Model file for the job. Use its own axes, mm. Face numbers are marked on the shaded views. A direction names the side the tool comes from. Round coordinates to 2 decimals unless told otherwise and drop trailing zeros. Order: outer loops, then holes, each group sorted by start corner. A loop starts at its lowest first (then second) coordinate and runs counter-clockwise, first axis right, second up. Notation, with made-up numbers: (67, -33.5) -> (119, -33.5) arc R21 ccw to (119, -11.5) -> close; hole circle Ø10 at (-18, 3). An arc over 180 degrees is marked (long way). Use CSV: the item, a comma, the result in double quotes.
Autodesk Inventor part; units mm, degrees
ref_plane "Work Plane1" through (-7, 0, 0) normal (-1, 0, 0) x (0, 0, 1)
ref_plane "Work Plane2" through (-7, 0, -17.9) normal (0, -1, 0) x (1, 0, 0)
ref_plane "YZ Plane" through (0, 0, 0) normal (1, 0, 0) x (0, 1, 0)
sketch "Sketch1" plane through (0, 0, 0) normal (1, 0, 0) x (0, 1, 0)
  arc A0 (-3.4641, 2) -> (3.4641, 2) centre (0, 0) ccw
  arc A1 (-5.1962, 3) -> (5.1962, 3) centre (0, 0) ccw
  arc A2 (5.1962, 3) -> (3.4641, 2) centre (4.3301, 2.5) ccw
  arc A3 (-3.4641, 2) -> (-5.1962, 3) centre (-4.3301, 2.5) ccw
  dimension "d0" = 8
  dimension "d1" = 12
  dimension "d2" = 2.5
extrude "Extrusion1" add sketch "Sketch1" along normal blind 16
sketch "Sketch4" plane through (16, 0, 0) normal (1, 0, 0) x (0, 0, -1)
  point P0 (0, 0)
sketch "Sketch5" plane through (16, 0, 0) normal (1, 0, 0) x (0, 0, -1)
  line L0 (-6.2503, -10.1933) -> (7.7655, -10.1933)
  line L1 (7.7655, -10.1933) -> (7.7655, 0)
  line L2 (7.7655, 0) -> (-6.2503, 0)
  line L3 (-6.2503, 0) -> (-6.2503, -10.1933)
  point P0 (0, 0)
extrude "Extrusion4" cut sketch "Sketch5" against normal blind 3
ref_plane "Work Plane1" through (-7, 0, 0) normal (-1, 0, 0) x (0, 0, 1)
sketch "Sketch9" plane through (-7, 0, 0) normal (-1, 0, 0) x (0, 0, 1)
  line L0 (-17.9, 10) -> (-11.4, 10)
  line L1 (-11.4, 10) -> (-11.4, -10)
  line L2 (-11.4, -10) -> (-17.9, -10)
  line L3 (-17.9, -10) -> (-17.9, 10)
  point P0 (0, 0)
  point P1 (-17.9, 0)
  dimension "d34" = 11.4
  dimension "d35" = 6.5
  dimension "d36" = 20
extrude "Extrusion8" add sketch "Sketch9" along normal blind 5
ref_plane "Work Plane2" through (-7, 0, -17.9) normal (0, -1, 0) x (1, 0, 0)
sketch "Sketch10" plane through (-7, 0, -17.9) normal (0, -1, 0) x (1, 0, 0)
  line L0 (7, 11) -> (23, 11)
  line L1 (0, 0) -> (0, 6.5)
  line L2 (7, 11.9) -> (0, 6.5)
  line L3 (0, 0) -> (-5, 0)
  line L4 (0, 6.5) -> (0, 0)
  line L5 (0, 0) -> (15.4259, 11.9)
  line L6 (7, 11.9) -> (7, 20.9)
  line L7 (15.4259, 11.9) -> (7, 11.9)
  point P0 (7, 17.9)
extrude "Extrusion9" add sketch "Sketch10" along normal mid plane 8
sketch "Sketch11" plane through (0, 0, 0) normal (-1, 0, 0) x (0, 0, 1)
  line L0 (-6, -4) -> (-6, 0)
  line L1 (-6, -4) -> (-4.4721, -4)
  arc A0 (-6, 0) -> (3, -5.1962) centre (0, 0) ccw
  line L2 (-6, 4) -> (-6, 0)
  line L3 (-6, 4) -> (-4.4721, 4)
  arc A1 (3, 5.1962) -> (-6, 0) centre (0, 0) ccw
extrude "Extrusion10" add sketch "Sketch11" against normal blind 9.1
fillet "Fillet3" radius 2 2 edges at (4.55, 4, -4.4721) (4.55, -4, -4.4721)
properties part number "Roller_Spacer"
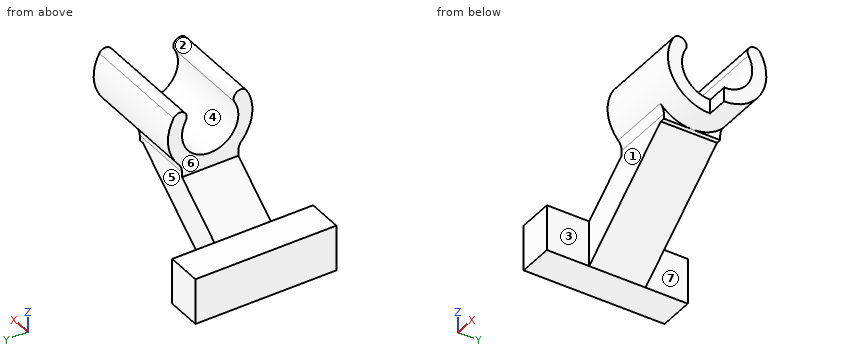
Q1. Cut at D-D (z = -7.5). Give the cut face in (x, y), plus the area to 3 significant figures.
From the geometry:
outline,"(-1.94, -4) -> (6.48, -4) -> (6.48, 4) -> (-1.94, 4) -> close"
area,"67.4 mm²"
Q2. Mould opens along Y. For the marked faces 1, 2, 3 and 4 say: +Y half, -Y half, draft (parallel to the pull), parting line (faces both ways), or undercut.
From the geometry:
face 1,"-Y half"
face 2,"undercut"
face 3,"draft"
face 4,"undercut"
Q3. Cut at A-A (z = 0). Give the cut face in (x, y).
From the geometry:
outline,"(0, -6) -> (13, -6) -> (13, -4) -> (0, -4) -> close; (0, 4) -> (16, 4) -> (16, 6) -> (0, 6) -> close"
Q4. Cut at B-B (y = 2.5). Give the cut face in (x, z), plus the area to 3 significant figures.
From the geometry:
outline,"(-12, -17.9) -> (-7, -17.9) -> (8.43, -6) -> (9.1, -6) -> (9.1, -5.45) -> (16, -5.45) -> (16, -3.12) -> (0, -3.12) -> (0, -6) -> (-7, -11.4) -> (-12, -11.4) -> close"
area,"148 mm²"
Q5. Which spindle directions (+Z, -Z, +X, -X, +Y, -Y) get a long thin tool onto all of the face, cutting with end or side? Do the marked faces 5, 6 and 7. Say none if no direction does.
From the geometry:
face 5,"-Z, +X, +Y"
face 6,"+Z, -X, +Y, -Y"
face 7,"+Z, -Z, +X, +Y"
Q6. Pin check, flat tips, straight feed: pin 1 (8 mm diameter, centred on x = 7, z = -4, fed in from +Y); pin 2 (10.5 mm diameter, centred on y = 0, z = 0, fed in from -X); pin 3 (2.5 mm diameter, centred on x = -10.5, y = -2.5, fed in from +Z); pin 4 (12 mm diameter, centred on x = 9, y = -3.5, fed in from +Z). Stop position of each tip, or through.
From the geometry:
pin 1,"stops at y = 6"
pin 2,"stops at x = 0"
pin 3,"stops at z = -11.4"
pin 4,"stops at z = 3.5"
Q7. Probe line 1 along Y through (x, z) = (5.5, 0); line 2 along Y through (x, z) = (-6.25, -16.25); line 3 along X through (y, z) = (4.25, 1.75). List the from-to ranges inside material, lowest first.
From the geometry:
line 1,"y = -6 to -4, 4 to 6"
line 2,"y = -4 to 4"
line 3,"x = 0 to 16"
Q8. Cut at C-C (x = 4.5). Give the cut face in (y, z).
From the geometry:
outline,"(-5.2, 3) arc R6 ccw to (-4.5, -3.97) arc R2 cw to (-4, -5.29) -> (-4, -9.03) -> (4, -9.03) -> (4, -5.29) arc R2 cw to (4.5, -3.97) arc R6 ccw to (5.2, 3) arc R1 ccw to (3.46, 2) arc R4 cw (long way) to (-3.46, 2) arc R1 ccw to start"
